Verification items for the finished model (mm, model axes). A direction names the side the tool comes from. Coordinates: 2 decimals unless noted, no trailing zeros. Order: outer loops, then holes, each group sorted by start corner. A loop starts at its lowest first (then second) coordinate and runs counter-clockwise, first axis right, second up.
Q1. Cross-section at A-A, the plane x = 0. Record the boundary of the cut face in (y, z), and give its area (3 significant figures).
Q2. Cross-section at B-B, the plane z = 0. Record the boundary of the cut face in (x, y), and give its area (3 significant figures).
Q3. Depth check by flat-ended pin: P1, Ø3, axis at y = -1, z = -12, coming from the -X side; P2, Ø2.5, axis at y = -2.5, z = -14.5, coming from the -X side; P3, Ø0.6, axis at x = -14.5, y = -3, coming from the -Z side. Enter the tip coordinate at first touch or a pass-through.
Q4. Set-up check for faces 4 (the flat face through (0, -4, 14)), 5 (the cylindrical face through (13.52, -1.97, 0.02)): record each of +Z, -Z, +X, -X, +Y, -Y from which the full face is reachable in a straight line by a thin tool's end or side.
Q5. Cross-section at D-D, the plane y = -5. Record the boundary of the cut face in (x, z).
Q6. Cross-section at C-C, the plane y = -2.5. Record the boundary of the cut face in (x, z).
Q7. Thickness scan on line 1 (Z direction, x = 0, y = -2.75); line 2 (Z direction, x = 0, y = -4.5); line 3 (X direction, y = -4.75, z = 5). Record the ranges inside material, lowest first.
Q8. Draft check along X on faces 1 (the flat face through (0, -4, -14)), 2 (the cylindrical face through (-4.01, -3.45, -18.06)), 3 (the flat face through (0, 0, -14)). Enter one of: pulls with the +X half, pulls with the -X half, needs draft (parallel to the pull), parting line crosses it, or undercut.
from build123d import *

# Parameters (mm, degrees)
F0_R            = 18.5
F0_R_2          = 15.5
F1_DEPTH        = 7
F3_DEPTH        = 4
F3_COPIES_COUNT = 4
F4_R            = 0.2
F5_T6_ANGLE     = 80.7189590371
F5_T12_ANGLE    = 80.7189590371
F5_T18_ANGLE    = 80.7189590371
F5_T24_ANGLE    = 80.7189590371


# Not quite as in the source:
# - a fillet or chamfer that OpenCascade refuses, or shapes differently, is made with other operations: its cross-section is extruded or revolved along the edge and cut away or added
# - a pattern or mirror of a feature is missing from the dataset's text; its kind, count and spacing are read off the source's solid


with BuildPart() as f1:
    # F0 (on Front) → F1 (new body)
    with BuildSketch(Plane.XZ):
        Circle(F0_R)
        Circle(F0_R_2, mode=Mode.SUBTRACT)
    extrude(amount=F1_DEPTH)

    # F2 (on Front) → F3 (join)
    with BuildSketch(Plane.XZ):
        with BuildLine():
            ThreePointArc((-2, 13.3704261489), (0, 13.5191824976), (2, 13.3704261489))
            Line((2, 13.3704261489), (2, 15.3704261489))
            ThreePointArc((2, 15.3704261489), (0, 15.5), (-2, 15.3704261489))
            Line((-2, 15.3704261489), (-2, 13.3704261489))
        make_face()
    f3 = extrude(amount=F3_DEPTH)

    # F3_copies: F3 ×4 about axis
    f3_copies_axis = Axis((0, 0, 0), (0, 1, 0))
    for i in range(1, F3_COPIES_COUNT):
        add(f3.rotate(f3_copies_axis, i * 360 / F3_COPIES_COUNT))

    # F4
    f4_edges = [f1.edges().sort_by_distance(p)[0] for p in [
        (2, -2, 13.370426),
        (-2, -2, 13.370426),
        (13.370426, -2, 2),
        (13.370426, -2, -2),
        (2, -2, -13.370426),
        (-2, -2, -13.370426),
        (-13.370426, -2, 2),
        (-13.370426, -2, -2),
    ]]
    fillet(f4_edges, radius=F4_R)

    # F5: fillet of radius 0.3 on 5 edges, made by hand

    # F5_s1 → F5_t2 (revolve, cut)
    with BuildSketch(Plane.XY):
        with BuildLine():
            ThreePointArc((15.5, -6.7), (15.5878679656, -6.9121320344), (15.8, -7))
            Line((15.8, -7), (15.5, -7))
            Line((15.5, -7), (15.5, -6.7))
        make_face()
    revolve(axis=Axis((0, -7, 0), (0, -1, 0)), mode=Mode.SUBTRACT)


with BuildPart() as f5_tool4:
    # F5_s5 → F5_t6 (revolve)
    with BuildSketch(Plane(origin=(0, 0, 0), x_dir=(0, 1, 0), z_dir=(0.080903842, 0, -0.9967219112))):
        with BuildLine():
            ThreePointArc((0, 15.8), (-0.0878679656, 15.5878679656), (-0.3, 15.5))
            Line((-0.3, 15.5), (0, 15.5))
            Line((0, 15.5), (0, 15.8))
        make_face()
    revolve(axis=Axis((0, 0, 0), (0, -1, 0)), revolution_arc=F5_T6_ANGLE)

    split(bisect_by=Plane.XY.offset(2), keep=Keep.TOP)

    split(bisect_by=Plane.YZ.offset(2), keep=Keep.TOP)


with BuildPart() as f1_1:
    add(f1.part)

    # F5_t3: cut F5_tool4
    add(f5_tool4.part, mode=Mode.SUBTRACT)


with BuildPart() as f5_tool10:
    # F5_s11 → F5_t12 (revolve)
    with BuildSketch(Plane(origin=(0, 0, 0), x_dir=(0, 1, 0), z_dir=(-0.9967219112, 0, -0.080903842))):
        with BuildLine():
            ThreePointArc((0, 15.8), (-0.0878679656, 15.5878679656), (-0.3, 15.5))
            Line((-0.3, 15.5), (0, 15.5))
            Line((0, 15.5), (0, 15.8))
        make_face()
    revolve(axis=Axis((0, 0, 0), (0, -1, 0)), revolution_arc=F5_T12_ANGLE)

    split(bisect_by=Plane.XY.offset(-2), keep=Keep.BOTTOM)

    split(bisect_by=Plane.YZ.offset(2), keep=Keep.TOP)


with BuildPart() as f1_2:
    add(f1_1.part)

    # F5_t9: cut F5_tool10
    add(f5_tool10.part, mode=Mode.SUBTRACT)


with BuildPart() as f5_tool16:
    # F5_s17 → F5_t18 (revolve)
    with BuildSketch(Plane(origin=(0, 0, 0), x_dir=(0, 1, 0), z_dir=(0.9967219112, 0, 0.080903842))):
        with BuildLine():
            ThreePointArc((0, 15.8), (-0.0878679656, 15.5878679656), (-0.3, 15.5))
            Line((-0.3, 15.5), (0, 15.5))
            Line((0, 15.5), (0, 15.8))
        make_face()
    revolve(axis=Axis((0, 0, 0), (0, -1, 0)), revolution_arc=F5_T18_ANGLE)

    split(bisect_by=Plane.YZ.offset(-2), keep=Keep.BOTTOM)

    split(bisect_by=Plane.XY.offset(2), keep=Keep.TOP)


with BuildPart() as f1_3:
    add(f1_2.part)

    # F5_t15: cut F5_tool16
    add(f5_tool16.part, mode=Mode.SUBTRACT)


with BuildPart() as f5_tool22:
    # F5_s23 → F5_t24 (revolve)
    with BuildSketch(Plane(origin=(0, 0, 0), x_dir=(0, 1, 0), z_dir=(-0.080903842, 0, 0.9967219112))):
        with BuildLine():
            ThreePointArc((0, 15.8), (-0.0878679656, 15.5878679656), (-0.3, 15.5))
            Line((-0.3, 15.5), (0, 15.5))
            Line((0, 15.5), (0, 15.8))
        make_face()
    revolve(axis=Axis((0, 0, 0), (0, -1, 0)), revolution_arc=F5_T24_ANGLE)

    split(bisect_by=Plane.YZ.offset(-2), keep=Keep.BOTTOM)

    split(bisect_by=Plane.XY.offset(-2), keep=Keep.BOTTOM)


with BuildPart() as f1_4:
    add(f1_3.part)

    # F5_t21: cut F5_tool22
    add(f5_tool22.part, mode=Mode.SUBTRACT)


solid = f1_4.part
Check values:
1. outline: (-7, -18.5) - (0, -18.5) - (0, -13.52) - (-4, -13.52) - (-4, -15.5) - (-6.7, -15.5) arc R0.3 ccw to (-7, -15.8) - close; (-7, 15.8) arc R0.3 ccw to (-6.7, 15.5) - (-4, 15.5) - (-4, 13.52) - (0, 13.52) - (0, 18.5) - (-7, 18.5) - close
1. area: 57.8 mm2
2. outline: (-18.5, -7) - (-15.8, -7) arc R0.3 ccw to (-15.5, -6.7) - (-15.5, -4) - (-13.52, -4) - (-13.52, 0) - (-18.5, 0) - close; (13.52, -4) - (15.5, -4) - (15.5, -6.7) arc R0.3 ccw to (15.8, -7) - (18.5, -7) - (18.5, 0) - (13.52, 0) - close
2. area: 57.8 mm2
3. P1: stops at x = -15.23
3. P2: stops at x = -12.91
3. P3: stops at z = -11.86
4. face 4: -Y
4. face 5: +Y, -Y
5. outline: circle Ø37 at (0, 0); hole circle Ø31 at (0, 0)
6. outline: circle Ø37 at (0, 0); hole (-15.37, -2) arc R15.5 ccw to (-2, -15.37) - (-2, -13.6) arc R0.2 cw to (-1.77, -13.4) arc R13.52 ccw to (1.77, -13.4) arc R0.2 cw to (2, -13.6) - (2, -15.37) arc R15.5 ccw to (15.37, -2) - (13.6, -2) arc R0.2 cw to (13.4, -1.77) arc R13.52 ccw to (13.4, 1.77) arc R0.2 cw to (13.6, 2) - (15.37, 2) arc R15.5 ccw to (2, 15.37) - (2, 13.6) arc R0.2 cw to (1.77, 13.4) arc R13.52 ccw to (-1.77, 13.4) arc R0.2 cw to (-2, 13.6) - (-2, 15.37) arc R15.5 ccw to (-15.37, 2) - (-13.6, 2) arc R0.2 cw to (-13.4, 1.77) arc R13.52 ccw to (-13.4, -1.77) arc R0.2 cw to (-13.6, -2) - close
7. line 1: z = -18.5 to -13.52, 13.52 to 18.5
7. line 2: z = -18.5 to -15.5, 15.5 to 18.5
7. line 3: x = -17.81 to -14.67, 14.67 to 17.81
8. face 1: undercut
8. face 2: parting line crosses it
8. face 3: needs draft
